Autodesk Inventor part; units mm, degrees
ref_plane "YZ Plane" through (0, 0, 0) normal (1, 0, 0) x (0, 1, 0)
ref_plane "XZ Plane" through (0, 0, 0) normal (0, 1, 0) x (-1, 0, 0)
ref_plane "XY Plane" through (0, 0, 0) normal (0, 0, 1) x (1, 0, 0)
sketch "Szkic1" plane through (0, 0, 0) normal (1, 0, 0) x (0, 1, 0)
  line L0 (0, 0) -> (12, 0)
  line L1 (12, 0) -> (12, 1.5)
  line L2 (12, 1.5) -> (1.5, 1.5)
  line L3 (1.5, 1.5) -> (1.5, 12)
  line L4 (1.5, 12) -> (0, 12)
  line L5 (0, 12) -> (0, 0)
  dimension "d0" = 12
  dimension "d1" = 1.5
  dimension "d2" = 10.5
  dimension "d3" = 10.5
extrude "Wyciągnięcie proste1" add sketch "Szkic1" along normal mid plane 170
sketch "Szkic2" plane through (-85, 0, 0) normal (0, -1, 0) x (1, 0, 0)
  line L0 (0, 12) -> (170, 12)
  line L1 (85, 0) -> (85, 6.75) construction
  dimension "d6" = 5.25
hole "Otwór1" at (0, 0, 6.75) direction (0, 1, 0) diameter 3.5 end through all
sketch "Szkic3" plane through (-85, 1.5, 1.5) normal (0, 0, 1) x (1, 0, 0)
  line L0 (0, 10.5) -> (170, 10.5) construction
  line L1 (85, 10.5) -> (85, 5.25) construction
  point P0 (85, -1.5)
  dimension "d14" = 5.25
hole "Otwór2" at (0, 6.75, 1.5) direction (0, 0, -1) diameter 3.5 end through all
sketch "Szkic4" plane through (-85, 1.5, 1.5) normal (0, 0, 1) x (1, 0, 0)
  line L0 (170, 10.5) -> (170, 0)
  line L1 (0, 10.5) -> (170, 10.5)
  point P0 (85, -1.5)
  point P1 (164.75, 5.25)
  dimension "d22" = 5.25
  dimension "d23" = 5.25
hole "Otwór3" at (79.75, 6.75, 1.5) direction (0, 0, -1) diameter 3.5 end through all
mirror "Odbij1" about plane through (0, 0, 0) normal (1, 0, 0) of "Otwór3"
pattern_linear "Szyk prostokątny1" count 3 spacing 14.5 along (1, 0, 0) of "Otwór2" first direction both ways yes
sketch "Szkic5" plane through (-85, 1.5, 12) normal (0, 1, 0) x (1, 0, 0)
  line L0 (0, 0) -> (170, 0) construction
  circle A0 centre (85, 5.25) radius 1.75 construction
  line L1 (85, 0) -> (85, 5.25) construction
  line L2 (120, 5.25) -> (50, 5.25) construction
  point P0 (85, 12)
  dimension "d34" = 70
hole "Otwór4" at (-35, 1.5, 6.75) at (35, 1.5, 6.75) direction (0, -1, 0) diameter 3.5 end through all
properties part number "bepf_platforma_rama_bok_dlugi" material "Aluminium 6061"
The model under review builds one solid part; all positions refer to its coordinate system, in mm. Round coordinates to 2 decimals unless told otherwise and drop trailing zeros. Loops run counter-clockwise (first coordinate to the right, second up) from the corner with the lowest first, then second, coordinate; pieces in that order, holes last.
Item 1: Take a section at C-C (y = 6.75). Write out the cut boundary in (x, z), then the cut area to 3 significant figures.
Determined:
outline: (-85, 0) - (-81.5, 0) - (-81.5, 1.5) - (-85, 1.5) - close; (-78, 0) - (-16.25, 0) - (-16.25, 1.5) - (-78, 1.5) - close; (-12.75, 0) - (-1.75, 0) - (-1.75, 1.5) - (-12.75, 1.5) - close; (1.75, 0) - (12.75, 0) - (12.75, 1.5) - (1.75, 1.5) - close; (16.25, 0) - (78, 0) - (78, 1.5) - (16.25, 1.5) - close; (81.5, 0) - (85, 0) - (85, 1.5) - (81.5, 1.5) - close
area: 229 mm2
Item 2: For line 1 (X direction, y = 6.75, z = 0.75); line 2 (Z direction, x = 0, y = 0.9), list the stretches that pass through material, from the lowest coordinate up.
Determined:
line 1: x = -85 to -81.5, -78 to -16.25, -12.75 to -1.75, 1.75 to 12.75, 16.25 to 78, 81.5 to 85
line 2: z = 0 to 5, 8.5 to 12
Item 3: Clearance check with flat-ended pins moving along their axes: pin 1 Ø5 at (x, z) = (6, 8) entering from +Y; pin 2 Ø4.5 at (x, y) = (0, 6.75) entering from +Z. State where each tip first meets the part, or that it passes through.
Determined:
pin 1: stops at y = 1.5
pin 2: stops at z = 1.5
Item 4: Take a section at D-D (x = 79.75). Write out the cut boundary in (y, z).
Determined:
outline: (0, 0) - (5, 0) - (5, 1.5) - (1.5, 1.5) - (1.5, 12) - (0, 12) - close; (8.5, 0) - (12, 0) - (12, 1.5) - (8.5, 1.5) - close
Item 5: Take a section at A-A (z = 6.75). Write out the cut boundary in (x, y).
Determined:
outline: (-85, 0) - (-36.75, 0) - (-36.75, 1.5) - (-85, 1.5) - close; (-33.25, 0) - (-1.75, 0) - (-1.75, 1.5) - (-33.25, 1.5) - close; (1.75, 0) - (33.25, 0) - (33.25, 1.5) - (1.75, 1.5) - close; (36.75, 0) - (85, 0) - (85, 1.5) - (36.75, 1.5) - close
Item 6: Take a section at B-B (x = 0). Write out the cut boundary in (y, z), then the cut area to 4 significant figures.
Determined:
outline: (0, 0) - (5, 0) - (5, 1.5) - (1.5, 1.5) - (1.5, 5) - (0, 5) - close; (0, 8.5) - (1.5, 8.5) - (1.5, 12) - (0, 12) - close; (8.5, 0) - (12, 0) - (12, 1.5) - (8.5, 1.5) - close
area: 23.25 mm2
Item 7: Mouldability with a two-part tool opening along Y and no side actions: class faces 1 (the face through (-1, 1.5, 4)), 2 (the face through (-16.235, 6.978, 0.74)), 3 (the face through (-1, 9, 1.5)) as released by +Y, released by -Y, zero draft, split by the parting line, or undercut.
Determined:
face 1: released by +Y
face 2: undercut
face 3: zero draft
